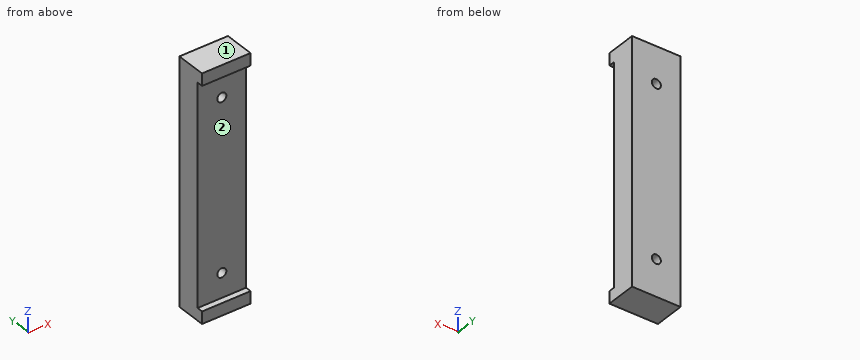
Autodesk Inventor part; units mm, degrees
ref_plane "YZ Plane" through (0, 0, 0) normal (1, 0, 0) x (0, 1, 0)
ref_plane "XZ Plane" through (0, 0, 0) normal (0, 1, 0) x (-1, 0, 0)
sketch "Sketch1" plane through (0, 0, 0) normal (0, 1, 0) x (-1, 0, 0)
  line L0 (25.4, 127) -> (-25.4, 127)
  line L1 (-25.4, 127) -> (-25.4, -127)
  line L2 (-25.4, -127) -> (25.4, -127)
  line L3 (25.4, -127) -> (25.4, 127)
  line L4 (25.4, 127) -> (-25.4, -127) construction
  line L5 (-25.4, 127) -> (25.4, -127) construction
  point P0 (0, 0)
  dimension "d0" = 50.8
  dimension "d1" = 254
extrude "Extrusion1" add sketch "Sketch1" along normal blind 25.4
sketch "Sketch2" plane through (0, 0, 0) normal (0, -1, 0) x (1, 0, 0)
  line L0 (-25.4, 127) -> (-25.4, 114.3)
  line L1 (-25.4, 114.3) -> (25.4, 114.3)
  line L2 (25.4, 114.3) -> (25.4, 127)
  line L3 (25.4, 127) -> (-25.4, 127)
  line L4 (-25.4, 127) -> (25.4, 114.3) construction
  line L5 (-25.4, 114.3) -> (25.4, 127) construction
  line L6 (-25.4, 127) -> (25.4, 127)
  point P0 (0, 0)
  point P1 (0, 120.65)
  dimension "d4" = 12.7
  dimension "d5" = 25.4
  dimension "d6" = 0
extrude "Extrusion2" add sketch "Sketch2" along normal blind 6.35
mirror "Mirror1" about plane through (0, 0, 0) normal (0, 0, 1) of "Extrusion2"
sketch "Sketch3" plane through (0, 25.4, 0) normal (0, 1, 0) x (1, 0, 0)
  circle A0 centre (0, -88.9) radius 4.7625
  line L0 (-25.4, -127) -> (25.4, -127)
  point P0 (0, 0)
  dimension "d9" = 9.525
  dimension "d10" = 38.1
extrude "Extrusion3" cut sketch "Sketch3" against normal through all
mirror "Mirror2" about plane through (0, 0, 0) normal (0, 0, 1) of "Extrusion3"
properties part number "BandSawJigTop" material "LCP Plastic"
Can you work these out from the model? Positions are in its coordinate system, mm. Face numbers are marked on the shaded views. A direction names the side the tool comes from. Give positions to 0.01 mm unless a question says otherwise; leave off trailing zeros. Loops run counter-clockwise (first coordinate to the right, second up) from the corner with the lowest first, then second, coordinate; pieces in that order, holes last. Notation, with made-up numbers: M -13.5,41.25 L 11.5,41.25 A8 cw 11.5,45.25 Z; hole C 53,49 d11. An arc over 180 degrees is marked long. One line per item, written item: value.
(1) Will these pins go through, and if not, where does the flat tip stop? pin 1 (5 mm diameter, centred on x = 15.5, z = 89.5, fed in from -Y); pin 2 (5.5 mm diameter, centred on x = 0, z = -88.9, fed in from -Y).
Returned:
pin 1: y = 0
pin 2: through
(2) Suppose I cut it at B-B on z = 88.9. List the corners of the cut face in (x, y) for me.
Returned:
outline: M -25.4,0 L -4.76,0 L -4.76,25.4 L -25.4,25.4 Z; M 4.76,0 L 25.4,0 L 25.4,25.4 L 4.76,25.4 Z
(3) Suppose I cut it at C-C on x = 16. List the corners of the cut face in (y, z) for me.
Returned:
outline: M -6.35,-127 L 25.4,-127 L 25.4,127 L -6.35,127 L -6.35,114.3 L 0,114.3 L 0,-114.3 L -6.35,-114.3 Z
(4) I need wall thicknesses on line 1 (Z direction, x = 0, y = 17.5); line 2 (X direction, y = 9.5, z = -88.9); line 3 (Y direction, x = -7, z = -31). Which ranges of each line are inside material? Lowest first, please.
Returned:
line 1: -127 to -93.66, -84.14 to 84.14, 93.66 to 127
line 2: -25.4 to -4.76, 4.76 to 25.4
line 3: 0 to 25.4
(5) Which directions (+Z, -Z, +X, -X, +Y, -Y) give clear straight access to the entire face, cutting with the end or side of a thin tool? Please do the marked faces 1 and 2.
Returned:
face 1: +Z, +X, -X, +Y, -Y
face 2: +X, -X, -Y
(6) Suppose I cut it at D-D on z = 33.5. List the corners of the cut face in (x, y) for me.
Returned:
outline: M -25.4,0 L 25.4,0 L 25.4,25.4 L -25.4,25.4 Z
(7) Suppose I cut it at A-A on x = 0. List the corners of the cut face in (y, z) for me, plus the area to 3 significant figures.
Returned:
outline: M -6.35,-127 L 25.4,-127 L 25.4,-93.66 L 0,-93.66 L 0,-114.3 L -6.35,-114.3 Z; M -6.35,114.3 L 0,114.3 L 0,93.66 L 25.4,93.66 L 25.4,127 L -6.35,127 Z; M 0,-84.14 L 25.4,-84.14 L 25.4,84.14 L 0,84.14 Z
area: 6,130 mm^2
